```python
from build123d import *

# Parameters (mm, degrees)
SKETCH1_R                               = 4
BUMPER_LINK_DEPTH                       = 3
SKETCH3_R                               = 8.125
BEARING_BLOCK_DEPTH                     = 7
BEARING_START                           = -2
SKETCH4_R                               = 8.125
SKETCH4_R_2                             = 5
BEARING_END_FLANGE_DEPTH                = 2
MIRRORED_BEARING_BLOCK_CONNECTION_DEPTH = 3


with BuildPart() as part:
    # Sketch1 → Bumper link (new body)
    with BuildSketch(Plane.XY):
        with BuildLine():
            Line((-12.098962679, -61.104930733), (-12.098962679, -63.762456748))
            ThreePointArc((-12.098962679, -63.762456748), (-11.741328645, -64.734567853), (-10.838962679, -65.24313227))
            Line((-10.838962679, -65.24313227), (10.838962679, -68.75686773))
            ThreePointArc((10.838962679, -68.75686773), (12.051073784, -68.418558175), (12.578962679, -67.276192209))
            Line((12.578962679, -67.276192209), (12.578962679, -64.618666193))
            ThreePointArc((12.578962679, -64.618666193), (13.046119656, -63.530900001), (14.156609733, -63.12067723))
            Line((14.156609733, -63.12067723), (52.741176488, -65.12067723))
            ThreePointArc((52.741176488, -65.12067723), (56.442810076, -63.753267994), (58, -60.127380685))
            Line((58, -60.127380685), (58, 37.87932277))
            ThreePointArc((58, 37.87932277), (56.535533906, 41.414856676), (53, 42.87932277))
            Line((53, 42.87932277), (48, 42.87932277))
            ThreePointArc((48, 42.87932277), (46.585786438, 43.465109208), (46, 44.87932277))
            Line((46, 44.87932277), (46, 54.964915964))
            ThreePointArc((46, 54.964915964), (44.937003937, 58.047122965), (42.2, 59.818780404))
            Line((42.2, 59.818780404), (-21.754442807, 75.629961849))
            ThreePointArc((-21.754442807, 75.629961849), (-26.508147155, 75.641290323), (-30.729965317, 73.456322411))
            Line((-30.729965317, 73.456322411), (-54.135467109, 53.028717314))
            ThreePointArc((-54.135467109, 53.028717314), (-57.221318402, 48.074910074), (-57.01624643, 42.242189451))
            Line((-57.01624643, 42.242189451), (-27.78932032, -42.733634568))
            ThreePointArc((-27.78932032, -42.733634568), (-22.022249502, -52.703383692), (-12.923793734, -59.765473046))
            ThreePointArc((-12.923793734, -59.765473046), (-12.321709099, -60.318404642), (-12.098962679, -61.104930733))
        make_face()
        with Locations((0, -59)):
            Circle(SKETCH1_R, mode=Mode.SUBTRACT)
        with Locations((-37.924468972, 45.196622144)):
            Circle(SKETCH1_R, mode=Mode.SUBTRACT)
        with Locations((39.478705775, 43.845544703)):
            Circle(SKETCH1_R, mode=Mode.SUBTRACT)
        with BuildLine():
            Line((33.5, 31.124748995), (33.5, -31.124748995))
            ThreePointArc((33.5, -31.124748995), (32.451435925, -35.582528136), (29.525641026, -39.105453865))
            ThreePointArc((29.525641026, -39.105453865), (10.554762126, -47.849733505), (-10.33433455, -47.897823848))
            ThreePointArc((-10.33433455, -47.897823848), (-14.864224576, -45.601026517), (-17.681588514, -41.375196178))
            Line((-17.681588514, -41.375196178), (-39.391489139, 21.745252689))
            ThreePointArc((-39.391489139, 21.745252689), (-39.769582846, 26.810055426), (-37.610876362, 31.407355497))
            ThreePointArc((-37.610876362, 31.407355497), (-5.581929526, 48.681023641), (29.525641026, 39.105453865))
            ThreePointArc((29.525641026, 39.105453865), (32.451435925, 35.582528136), (33.5, 31.124748995))
        make_face(mode=Mode.SUBTRACT)
    extrude(amount=BUMPER_LINK_DEPTH)

    # Sketch3 → Bearing block (add)
    with BuildSketch(Plane.ZY.offset(-33.5)):
        with BuildLine():
            Line((-17, 16.125), (0, 16.125))
            Line((0, 16.125), (0, -16.125))
            Line((0, -16.125), (-17, -16.125))
            ThreePointArc((-17, -16.125), (-33.125, 0), (-17, 16.125))
        make_face()
        with Locations(Location((-17, 0, 0), (0, 0, 270))):
            Circle(SKETCH3_R, mode=Mode.SUBTRACT)
    bearing_block = extrude(amount=-BEARING_BLOCK_DEPTH)

    # Sketch4 → Bearing end flange (add)
    with BuildSketch(Plane(origin=(40.5, 0, 0), x_dir=(0, 0, -1), z_dir=(1, 0, 0)).offset(BEARING_START)):
        with Locations(Location((17, 0, 0), (0, 0, 270))):
            Circle(SKETCH4_R)
        with Locations(Location((17, 0, 0), (0, 0, 90))):
            Circle(SKETCH4_R_2, mode=Mode.SUBTRACT)
    bearing_end_flange = extrude(amount=BEARING_END_FLANGE_DEPTH)

    # Mirror1: Bearing block, Bearing end flange across plane
    add(bearing_block.mirror(Plane(origin=(0, 0, 0), x_dir=(0, 0, 1), z_dir=(1, 0, 0))))
    add(bearing_end_flange.mirror(Plane(origin=(0, 0, 0), x_dir=(0, 0, 1), z_dir=(1, 0, 0))))

    # Sketch6 → Mirrored bearing block connection (add)
    with BuildSketch(Plane.XY):
        Polygon((-37.458436863, 16.125), (-33.5, 4.616043054), (-33.5, 16.125), align=None)
        Polygon((-40.5, -16.125), (-36.941200933, -16.125), (-40.5, -5.777969932), align=None)
    extrude(amount=MIRRORED_BEARING_BLOCK_CONNECTION_DEPTH)


solid = part.part
```
Verification items for the finished model (mm, model axes). A direction names the side the tool comes from. Round coordinates to 2 decimals unless told otherwise and drop trailing zeros. Write each loop counter-clockwise with the first axis right and the second up, starting at its lowest first coordinate (ties: lowest second). Pieces come first, ordered by that corner, then holes. Notation, with made-up numbers: (-12.75, 49) - (36.25, 49) arc R11 ccw to (36.25, 53) - close; hole circle Ø5 at (88.25, 45). An arc over 180 degrees is marked (long way). Answer as a JSON object with one key per item and string values. Group by question number.
Q1. Section check C-C, the plane x = 0. Enter the section's corners in (y, z), plus the area to 3 significant figures.
Q2. Go/stop test with flat-tipped pins: pin 1 Ø3.5 at (x, z) = (37, -7.5) entering from +Y (3 decimals); pin 2 Ø8 at (y, z) = (-3.5, -18) entering from +X; pin 3 Ø0.9 at (x, z) = (49.5, 2) entering from +Y. Record where each tip stops, or that it passes through.
Q3. Mould release check, pull along Y, two halves, no side actions. Record for faces 6 (the cylindrical face through (-35.965, 1.058, -8.944)), 7 (the cylindrical face through (-39.49, -1.08, -21.88)), 8 (the cylindrical face through (56.57, 41.38, 1.48)), 9 (the flat face through (33.179, -64.107, 1.479)): released by +Y, released by -Y, zero draft, split by the parting line, or undercut.
Q4. Tool access check on faces 1 (the flat face through (40.5, -3.4, -13.1)), 2 (the flat face through (-42.269, 63.386, 1.479)), 3 (the flat face through (51, 42.879, 1)), 4 (the cylindrical face through (-36.95, -0.35, -33.12)), 5 (the cylindrical face through (32.422, 35.64, 1.479)). Record the directions out of +Z, -Z, +X, -X, +Y, -Y that give a thin tool (end or side, any length) a straight path to the whole face; none if there is none.
Q5. Section check B-B, the plane y = 33. Enter the section's corners in (x, z), plus the area to 3 significant figures.
Q6. Thickness scan on line 1 (Y direction, x = 35, z = -17) (3 decimals); line 2 (Z direction, x = -39.5, y = 0) (3 decimals); line 3 (X direction, y = 44.5, z = 1.5). Record the ranges inside material, lowest first.
Q7. Section check A-A, the plane z = -3. Enter the section's corners in (x, y) (3 decimals).
Q8. Section check D-D, the plane y = 0. Give the number of separate pieces and of enclosed holes in the cut face, plus the area to 3 significant figures.
Found:
{
 "1": {"outline": "(-67, 0) - (-63, 0) - (-63, 3) - (-67, 3) - close; (-55, 0) - (-49, 0) - (-49, 3) - (-55, 3) - close; (49, 0) - (70.25, 0) - (70.25, 3) - (49, 3) - close", "area": "93.8 mm^2"},
 "2": {"pin 1": "stops at y = 16.125", "pin 2": "stops at x = 40.5", "pin 3": "stops at y = 42.88"},
 "3": {"face 6": "undercut", "face 7": "undercut", "face 8": "released by +Y", "face 9": "released by -Y"},
 "4": {"face 1": "-Z, +X, +Y, -Y", "face 2": "+Z, -Z, -X, +Y", "face 3": "+Z, -Z, +X, +Y", "face 4": "-Z, +X, -X", "face 5": "+Z, -Z"},
 "5": {"outline": "(-53.84, 0) - (-36.22, 0) - (-36.22, 3) - (-53.84, 3) - close; (33.32, 0) - (58, 0) - (58, 3) - (33.32, 3) - close", "area": "127 mm^2"},
 "6": {"line 1": "y = -16.125 to -8.125, 8.125 to 16.125", "line 2": "z = -33.125 to -22, -12 to 3", "line 3": "x = -57.51 to -41.86, -33.99 to -20.51, 20.51 to 35.53, 43.42 to 46.04"},
 "7": {"outline": "(-40.5, -16.125) - (-33.5, -16.125) - (-33.5, 16.125) - (-40.5, 16.125) - close; (33.5, -16.125) - (40.5, -16.125) - (40.5, 16.125) - (33.5, 16.125) - close"},
 "8": {"separate pieces": "4", "enclosed holes": "0", "area": "366 mm^2"}
}
